Could you check a few things on this drawing? It's one solid part, dimensions in mm from its lowest x, y, z. Round coordinates to 2 decimals unless told otherwise and drop trailing zeros. Loops run counter-clockwise (first coordinate to the right, second up) from the corner with the lowest first, then second, coordinate; pieces in that order, holes last. Notation, with made-up numbers: M -10.75,79 L 17.25,79 A5 cw 17.25,83 Z; hole C 45.5,7.25 d2. An arc over 180 degrees is marked long. Put each result on its own line as item: value. Start each with the question number.
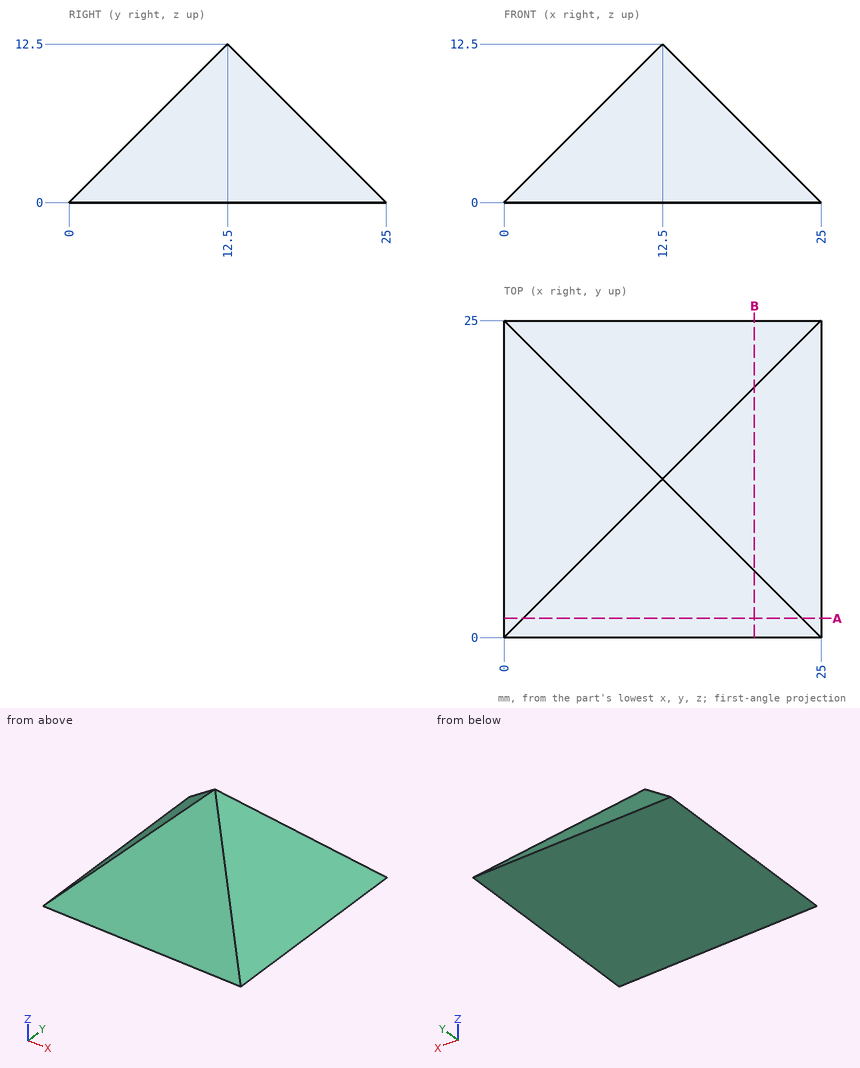
1) I'm going to push flat-ended pins straight in: P1, Ø6, axis at x = 20.5, y = 7, coming from the +Z side; P2, Ø2, axis at x = 11.5, y = 2.5, coming from the +Z side; P3, Ø4, axis at x = 18, z = 7.5, coming from the -Y side; P4, Ø12, axis at x = 4.5, y = 5, coming from the -Z side. Where does each tip first touch, or does it pass through?
2) Suppose I cut it at B-B (x = 19.75). Write out the boundary of the cut face in (y, z), plus the area to 3 significant figures.
3) Suppose I cut it at A-A (y = 1.5). Write out the boundary of the cut face in (x, z), plus the area to 4 significant figures.
4) If I drill on probe 1 along Y at (x, z) = (12, 2); probe 2 along Z at (x, y) = (15.75, 21.75); probe 3 along Z at (x, y) = (19.75, 10.25), over which ranges is the centre line in solid material (lowest first)? Write a range as from..to.
Results are:
1. P1: z = 7.46
1. P2: z = 3.5
1. P3: y = 5.5
1. P4: z = 0
2. outline: M 0,0 L 25,0 L 19.75,5.25 L 5.25,5.25 Z
2. area: 104 mm²
3. outline: M 0,0 L 25,0 L 23.5,1.5 L 1.5,1.5 Z
3. area: 35.25 mm²
4. probe 1: 2..23
4. probe 2: 0..3.25
4. probe 3: 0..5.25
